Check sheet for the modelled part. Datum: model origin and axes. Units: mm. Round coordinates to 2 decimals unless told otherwise and drop trailing zeros. Order: outer loops, then holes, each group sorted by start corner. A loop starts at its lowest first (then second) coordinate and runs counter-clockwise, first axis right, second up.
Q1. Scan lines: probe 1 along X at (y, z) = (-12.25, 228.6) (3 decimals); probe 2 along X at (y, z) = (-4.75, 33.5); probe 3 along X at (y, z) = (-10.25, 129). Record each from-to range of solid material in increasing order.
Q2. Cross-section at B-B on z = 189. Record the cut outline in (x, y), then the cut area to 3 significant figures.
Q3. Cross-section at C-C on z = 130. Record the cut outline in (x, y).
Q4. Cross-section at A-A on x = -88.9. Record the cut outline in (y, z) (3 decimals), then the cut area to 3 significant figures.
Q5. Cross-section at D-D on y = -20.25. Give the number of separate pieces and of enclosed holes in the cut face, then the cut area to 3 significant figures.
Q6. Mould release check, pull along X, two halves, no side actions. Record for faces 1 (the cylindrical face through (-80.11, -12.88, 21.2)), 2 (the flat face through (-114.3, -13, 131)), 3 (the flat face through (-71, 0, 135)): +X half, -X half, draft (parallel to the pull), parting line (faces both ways), or undercut.
Q7. Depth check by flat-ended pin: P1, Ø2, axis at y = -4.5, z = 84, coming from the +X side. Enter the tip coordinate at first touch or a pass-through.
from build123d import *

# Parameters (mm, degrees)
F0_W     = 114.3
F0_H     = 266.7
F1_DEPTH = 25.4
F2_R     = 3.175
F2_R_2   = 6.35
F2_R_3   = 9.525
F2_R_4   = 12.7
F2_R_5   = 15.875
F2_R_6   = 19.05
F3_DEPTH = 25.4
F5_DEPTH = 25.4


with BuildPart() as f1:
    # F0 (on Front) → F1 (new body)
    with BuildSketch(Plane.XZ):
        with Locations((-57.15, 133.35)):
            Rectangle(F0_W, F0_H)
    extrude(amount=F1_DEPTH)

    # F2 (on face) → F3 (cut)
    with BuildSketch(Plane.XZ.offset(25.4)):
        with BuildLine():
            ThreePointArc((-25.4, 57.15), (-44.45, 38.1), (-25.4, 19.05))
            Line((-25.4, 19.05), (-25.4, 38.1))
            Line((-25.4, 38.1), (-25.4, 57.15))
        make_face()
        with BuildLine():
            ThreePointArc((-25.4, 231.775), (-28.575, 228.6), (-25.4, 225.425))
            Line((-25.4, 225.425), (-25.4, 228.6))
            Line((-25.4, 228.6), (-25.4, 231.775))
        make_face()
        with BuildLine():
            Line((-25.4, 228.6), (-25.4, 225.425))
            ThreePointArc((-25.4, 225.425), (-23.154936, 226.354936), (-22.225, 228.6))
            ThreePointArc((-22.225, 228.6), (-23.154936, 230.845064), (-25.4, 231.775))
            Line((-25.4, 231.775), (-25.4, 228.6))
        make_face()
        with BuildLine():
            ThreePointArc((-25.4, 209.55), (-31.75, 203.2), (-25.4, 196.85))
            Line((-25.4, 196.85), (-25.4, 203.2))
            Line((-25.4, 203.2), (-25.4, 209.55))
        make_face()
        with BuildLine():
            Line((-25.4, 203.2), (-25.4, 196.85))
            ThreePointArc((-25.4, 196.85), (-20.909872, 198.709872), (-19.05, 203.2))
            ThreePointArc((-19.05, 203.2), (-20.909872, 207.690128), (-25.4, 209.55))
            Line((-25.4, 209.55), (-25.4, 203.2))
        make_face()
        with BuildLine():
            ThreePointArc((-25.4, 180.975), (-34.925, 171.45), (-25.4, 161.925))
            Line((-25.4, 161.925), (-25.4, 171.45))
            Line((-25.4, 171.45), (-25.4, 180.975))
        make_face()
        with BuildLine():
            Line((-25.4, 171.45), (-25.4, 161.925))
            ThreePointArc((-25.4, 161.925), (-18.664808, 164.714808), (-15.875, 171.45))
            ThreePointArc((-15.875, 171.45), (-18.664808, 178.185192), (-25.4, 180.975))
            Line((-25.4, 180.975), (-25.4, 171.45))
        make_face()
        with BuildLine():
            ThreePointArc((-25.4, 146.05), (-38.1, 133.35), (-25.4, 120.65))
            Line((-25.4, 120.65), (-25.4, 133.35))
            Line((-25.4, 133.35), (-25.4, 146.05))
        make_face()
        with BuildLine():
            Line((-25.4, 133.35), (-25.4, 120.65))
            ThreePointArc((-25.4, 120.65), (-16.419744, 124.369744), (-12.7, 133.35))
            ThreePointArc((-12.7, 133.35), (-16.419744, 142.330256), (-25.4, 146.05))
            Line((-25.4, 146.05), (-25.4, 133.35))
        make_face()
        with BuildLine():
            ThreePointArc((-25.4, 104.775), (-41.275, 88.9), (-25.4, 73.025))
            Line((-25.4, 73.025), (-25.4, 88.9))
            Line((-25.4, 88.9), (-25.4, 104.775))
        make_face()
        with BuildLine():
            Line((-25.4, 88.9), (-25.4, 73.025))
            ThreePointArc((-25.4, 73.025), (-14.17468, 77.67468), (-9.525, 88.9))
            ThreePointArc((-9.525, 88.9), (-14.17468, 100.12532), (-25.4, 104.775))
            Line((-25.4, 104.775), (-25.4, 88.9))
        make_face()
        with BuildLine():
            Line((-25.4, 38.1), (-25.4, 19.05))
            ThreePointArc((-25.4, 19.05), (-11.929616, 24.629616), (-6.35, 38.1))
            ThreePointArc((-6.35, 38.1), (-11.929616, 51.570384), (-25.4, 57.15))
            Line((-25.4, 57.15), (-25.4, 38.1))
        make_face()
        with Locations((-88.9, 228.6)):
            Circle(F2_R)
        with Locations((-88.9, 203.2)):
            Circle(F2_R_2)
        with Locations((-88.9, 171.45)):
            Circle(F2_R_3)
        with Locations((-88.9, 133.35)):
            Circle(F2_R_4)
        with Locations((-88.9, 88.9)):
            Circle(F2_R_5)
        with Locations((-88.9, 38.1)):
            Circle(F2_R_6)
    extrude(amount=-F3_DEPTH, mode=Mode.SUBTRACT)

    # F4 (on face) → F5 (cut)
    with BuildSketch(Plane.XZ.offset(25.4)):
        with BuildLine():
            ThreePointArc((-57.15, 247.65), (-76.2, 228.6), (-57.15, 209.55))
            Line((-57.15, 209.55), (-57.15, 228.6))
            Line((-57.15, 228.6), (-57.15, 247.65))
        make_face()
        with BuildLine():
            Line((-57.15, 228.6), (-57.15, 209.55))
            ThreePointArc((-57.15, 209.55), (-43.679616, 215.129616), (-38.1, 228.6))
            ThreePointArc((-38.1, 228.6), (-43.679616, 242.070384), (-57.15, 247.65))
            Line((-57.15, 247.65), (-57.15, 228.6))
        make_face()
        with BuildLine():
            ThreePointArc((-57.15, 193.675), (-73.025, 177.8), (-57.15, 161.925))
            Line((-57.15, 161.925), (-57.15, 177.8))
            Line((-57.15, 177.8), (-57.15, 193.675))
        make_face()
        with BuildLine():
            Line((-57.15, 177.8), (-57.15, 161.925))
            ThreePointArc((-57.15, 161.925), (-45.92468, 166.57468), (-41.275, 177.8))
            ThreePointArc((-41.275, 177.8), (-45.92468, 189.02532), (-57.15, 193.675))
            Line((-57.15, 193.675), (-57.15, 177.8))
        make_face()
        with BuildLine():
            ThreePointArc((-57.15, 146.05), (-69.85, 133.35), (-57.15, 120.65))
            Line((-57.15, 120.65), (-57.15, 133.35))
            Line((-57.15, 133.35), (-57.15, 146.05))
        make_face()
        with BuildLine():
            Line((-57.15, 133.35), (-57.15, 120.65))
            ThreePointArc((-57.15, 120.65), (-48.169744, 124.369744), (-44.45, 133.35))
            ThreePointArc((-44.45, 133.35), (-48.169744, 142.330256), (-57.15, 146.05))
            Line((-57.15, 146.05), (-57.15, 133.35))
        make_face()
        with BuildLine():
            ThreePointArc((-57.15, 104.775), (-66.675, 95.25), (-57.15, 85.725))
            Line((-57.15, 85.725), (-57.15, 95.25))
            Line((-57.15, 95.25), (-57.15, 104.775))
        make_face()
        with BuildLine():
            Line((-57.15, 95.25), (-57.15, 85.725))
            ThreePointArc((-57.15, 85.725), (-50.414808, 88.514808), (-47.625, 95.25))
            ThreePointArc((-47.625, 95.25), (-50.414808, 101.985192), (-57.15, 104.775))
            Line((-57.15, 104.775), (-57.15, 95.25))
        make_face()
        with BuildLine():
            ThreePointArc((-57.15, 69.85), (-63.5, 63.5), (-57.15, 57.15))
            Line((-57.15, 57.15), (-57.15, 63.5))
            Line((-57.15, 63.5), (-57.15, 69.85))
        make_face()
        with BuildLine():
            Line((-57.15, 63.5), (-57.15, 57.15))
            ThreePointArc((-57.15, 57.15), (-52.659872, 59.009872), (-50.8, 63.5))
            ThreePointArc((-50.8, 63.5), (-52.659872, 67.990128), (-57.15, 69.85))
            Line((-57.15, 69.85), (-57.15, 63.5))
        make_face()
        with BuildLine():
            ThreePointArc((-53.975, 38.1), (-54.904936, 40.345064), (-57.15, 41.275))
            ThreePointArc((-57.15, 41.275), (-59.395064, 35.854936), (-53.975, 38.1))
        make_face()
    extrude(amount=-F5_DEPTH, mode=Mode.SUBTRACT)


solid = f1.part
Results found:
1. probe 1: x = -114.3 to -92.075, -85.725 to -76.2, -38.1 to -28.575, -22.225 to 0
1. probe 2: x = -114.3 to -107.39, -70.41 to -43.89, -6.91 to 0
1. probe 3: x = -114.3 to -100.83, -76.97 to -69.08, -45.22 to -37.33, -13.47 to 0
2. outline: (-114.3, -25.4) - (-68.4, -25.4) - (-68.4, 0) - (-114.3, 0) - close; (-45.9, -25.4) - (0, -25.4) - (0, 0) - (-45.9, 0) - close
2. area: 2,330 mm2
3. outline: (-114.3, -25.4) - (-101.15, -25.4) - (-101.15, 0) - (-114.3, 0) - close; (-76.65, -25.4) - (-69.4, -25.4) - (-69.4, 0) - (-76.65, 0) - close; (-44.9, -25.4) - (-37.65, -25.4) - (-37.65, 0) - (-44.9, 0) - close; (-13.15, -25.4) - (0, -25.4) - (0, 0) - (-13.15, 0) - close
4. outline: (-25.4, 0) - (0, 0) - (0, 19.05) - (-25.4, 19.05) - close; (-25.4, 57.15) - (0, 57.15) - (0, 73.025) - (-25.4, 73.025) - close; (-25.4, 104.775) - (0, 104.775) - (0, 120.65) - (-25.4, 120.65) - close; (-25.4, 146.05) - (0, 146.05) - (0, 161.925) - (-25.4, 161.925) - close; (-25.4, 180.975) - (0, 180.975) - (0, 196.85) - (-25.4, 196.85) - close; (-25.4, 209.55) - (0, 209.55) - (0, 225.425) - (-25.4, 225.425) - close; (-25.4, 231.775) - (0, 231.775) - (0, 266.7) - (-25.4, 266.7) - close
4. area: 3,390 mm2
5. separate pieces: 1
5. enclosed holes: 18
5. area: 21,800 mm2
6. face 1: undercut
6. face 2: -X half
6. face 3: draft
7. P1: stops at x = 0
